from build123d import *

# Parameters (mm, degrees)
F0_R     = 2.75
F1_DEPTH = 0.4


with BuildPart() as f1:
    # F0 (on Top) → F1 (new body)
    with BuildSketch(Plane.XY):
        with BuildLine():
            Line((-5, 30), (-5, 0))
            ThreePointArc((-5, 0), (0, -5), (5, 0))
            Line((5, 0), (5, 30))
            Line((5, 30), (3.095048, 77.623802))
            ThreePointArc((3.095048, 77.623802), (0, 80.597523), (-3.095048, 77.623802))
            Line((-3.095048, 77.623802), (-5, 30))
        make_face()
        Circle(F0_R, mode=Mode.SUBTRACT)
    extrude(amount=F1_DEPTH)


solid = f1.part
Could you check a few things on this model? Use its own coordinates, in mm. Round coordinates to 2 decimals unless told otherwise and drop trailing zeros. Write each loop counter-clockwise with the first axis right and the second up, starting at its lowest first coordinate (ties: lowest second). Pieces come first, ordered by that corner, then holes. Notation, with made-up numbers: (19, -35.75) - (69, -35.75) arc R36 cw to (69, -1.75) - close; hole circle Ø5 at (8.25, 82). An arc over 180 degrees is marked (long way). Put each result on its own line as item: value. Start each with the question number.
(1) I want a section at B-B, the plane x = 0. Please give me the cut outline in (y, z).
(2) I want a section at D-D, the plane y = 46. Please give me the cut outline in (x, z), plus the area to 3 significant figures.
(3) I need wall thicknesses on probe 1 along Y at (x, z) = (0, 0.2); probe 2 along X at (y, z) = (2.5, 0.1); probe 3 along X at (y, z) = (0.5, 0.15). Which ranges of each line are inside material? Lowest first, please.
(4) Thinking about a two-plate mould opening in Y: for faces 1 (the flat face through (4.06, 53.48, 0.2)), 2 (the cylindrical face through (-0.596, -2.685, 0.197)), 3 (the flat face through (0, 38, 0)), which applies, released by +Y, released by -Y, zero draft, split by the parting line, or undercut?
(5) I want a section at A-A, the plane z = 0.25. Please give me the cut outline in (x, y).
(6) I want a section at C-C, the plane y = 1. Please give me the cut outline in (x, z), plus the area to 3 significant figures.
Here are the results:
1. outline: (-5, 0) - (-2.75, 0) - (-2.75, 0.4) - (-5, 0.4) - close; (2.75, 0) - (80.6, 0) - (80.6, 0.4) - (2.75, 0.4) - close
2. outline: (-4.36, 0) - (4.36, 0) - (4.36, 0.4) - (-4.36, 0.4) - close
2. area: 3.49 mm^2
3. probe 1: y = -5 to -2.75, 2.75 to 80.6
3. probe 2: x = -5 to -1.15, 1.15 to 5
3. probe 3: x = -5 to -2.7, 2.7 to 5
4. face 1: released by +Y
4. face 2: undercut
4. face 3: zero draft
5. outline: (-5, 0) arc R5 ccw to (5, 0) - (5, 30) - (3.1, 77.62) arc R3.1 ccw to (-3.1, 77.62) - (-5, 30) - close; hole circle Ø5.5 at (0, 0)
6. outline: (-5, 0) - (-2.56, 0) - (-2.56, 0.4) - (-5, 0.4) - close; (2.56, 0) - (5, 0) - (5, 0.4) - (2.56, 0.4) - close
6. area: 1.95 mm^2
